from build123d import *

# Parameters (mm, degrees)
F0_W     = 38
F0_H     = 38
F0_W_2   = 33
F0_H_2   = 33
F1_DEPTH = 962
F3_D     = 8.8


with BuildPart() as f1:
    # F0 (on Top) → F1 (new body)
    with BuildSketch(Plane.XY):
        Rectangle(F0_W, F0_H)
        Rectangle(F0_W_2, F0_H_2, mode=Mode.SUBTRACT)
    extrude(amount=F1_DEPTH)

    # F3 (through all)
    with Locations(Plane(origin=(-19, 0, 0), x_dir=(0, -1, 0), z_dir=(-1, 0, 0))):
        with Locations((0, 250), (0, 350), (0, 450), (0, 150), (0, 100), (0, 50), (0, 550), (0, 750), (0, 650), (0, 850)):
            Hole(F3_D / 2)


solid = f1.part
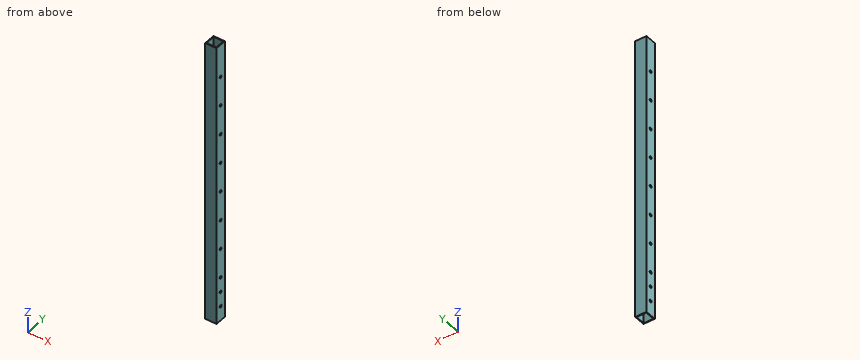
The listing builds one solid part. Answer for the finished solid, in the listing's coordinates (mm). Coordinates: 2 decimals unless noted, no trailing zeros. Loops run counter-clockwise (first coordinate to the right, second up) from the corner with the lowest first, then second, coordinate; pieces in that order, holes last. Notation, with made-up numbers: M 48,88 L 101,88 A15 cw 101,106 Z; hole C 52,72 d2. An arc over 180 degrees is marked long. Answer in a Markdown table with one row per item.
1) Find the intervals of material crossed by probe 1 along X at (y, z) = (3.5, 877); probe 2 along Y at (x, z) = (-17.9, 850), in increasing order.
Answers below:
| item | result |
|---|---|
| probe 1 | -19 to -16.5, 16.5 to 19 |
| probe 2 | -19 to -4.4, 4.4 to 19 |
2) Find section A-A (x = 0). Determine the outline of the cut face in (y, z).
Answers below:
| item | result |
|---|---|
| outline | M -19,0 L -16.5,0 L -16.5,962 L -19,962 Z; M 16.5,0 L 19,0 L 19,962 L 16.5,962 Z |
3) Find section B-B (z = 801). Determine the outline of the cut face in (x, y).
Answers below:
| item | result |
|---|---|
| outline | M -19,-19 L 19,-19 L 19,19 L -19,19 Z; hole M -16.5,-16.5 L 16.5,-16.5 L 16.5,16.5 L -16.5,16.5 Z |
